Could you check a few things on this model? Use its own coordinates, in mm. A direction names the side the tool comes from. Round coordinates to 2 decimals unless told otherwise and drop trailing zeros. Write each loop counter-clockwise with the first axis right and the second up, starting at its lowest first coordinate (ties: lowest second). Pieces come first, ordered by that corner, then holes. Notation, with made-up numbers: (76.25, 8) -> (93.25, 8) arc R16 ccw to (93.25, 15) -> close; hole circle Ø7 at (89, 83). An arc over 180 degrees is marked (long way). Return JSON: item names as keys, results as strings.
from build123d import *

# Parameters (mm, degrees)
F0_R        = 14.01
F1_DEPTH    = 8.2
F2_T1_DEPTH = 8.2
F3_C1_SIZE  = 1
F3_C2_SIZE  = 1
F3_C3_SIZE  = 1
F3_C4_SIZE  = 1
F3_C5_SIZE  = 1
F3_C6_SIZE  = 1
F3_C7_SIZE  = 1


# Not quite as in the source:
# - a fillet or chamfer that OpenCascade refuses, or shapes differently, is made with other operations: its cross-section is extruded or revolved along the edge and cut away or added


with BuildPart() as f1:
    # F0 (on Top) → F1 (new body)
    with BuildSketch(Plane.XY):
        with BuildLine():
            Line((-22.6979741071, -5), (-18.3303027798, -5))
            ThreePointArc((-18.3303027798, -5), (0, -19), (18.3303027798, -5))
            Line((18.3303027798, -5), (22.6979741071, -5))
            ThreePointArc((22.6979741071, -5), (58.01, 0), (22.6979741071, 5))
            Line((22.6979741071, 5), (18.3303027798, 5))
            ThreePointArc((18.3303027798, 5), (0, 19), (-18.3303027798, 5))
            Line((-18.3303027798, 5), (-22.6979741071, 5))
            ThreePointArc((-22.6979741071, 5), (-58.01, 0), (-22.6979741071, -5))
        make_face()
        with Locations((-40, 0)):
            Circle(F0_R, mode=Mode.SUBTRACT)
        Circle(F0_R, mode=Mode.SUBTRACT)
        with Locations((40, 0)):
            Circle(F0_R, mode=Mode.SUBTRACT)
    extrude(amount=F1_DEPTH)

    # F2: fillet of radius 5 on 8 edges, made by hand

    # F2_s2 → F2_t1 (join)
    with BuildSketch(Plane.XY):
        with BuildLine():
            ThreePointArc((-19.2765808806, -5), (-21.9350728052, -5.7653311007), (-23.7797141095, -7.8270317253))
            ThreePointArc((-23.7797141095, -7.8270317253), (-23.1793468046, -6.4362820074), (-22.6979741071, -5))
            Line((-22.6979741071, -5), (-19.2765808806, -5))
        make_face()
        with BuildLine():
            ThreePointArc((-21.8174242293, -5), (-19.1171156049, -5.7918729423), (-17.2721275148, -7.9166666667))
            ThreePointArc((-17.2721275148, -7.9166666667), (-17.8608509549, -6.4799693801), (-18.3303027798, -5))
            Line((-18.3303027798, -5), (-21.8174242293, -5))
        make_face()
        with BuildLine():
            ThreePointArc((17.2721275148, -7.9166666667), (19.1171156049, -5.7918729423), (21.8174242293, -5))
            Line((21.8174242293, -5), (18.3303027798, -5))
            ThreePointArc((18.3303027798, -5), (17.8608509549, -6.4799693801), (17.2721275148, -7.9166666667))
        make_face()
        with BuildLine():
            ThreePointArc((19.2765808806, -5), (21.9350728052, -5.7653311007), (23.7797141095, -7.8270317253))
            ThreePointArc((23.7797141095, -7.8270317253), (23.1793468046, -6.4362820074), (22.6979741071, -5))
            Line((22.6979741071, -5), (19.2765808806, -5))
        make_face()
        with BuildLine():
            ThreePointArc((21.8174242293, 5), (19.1171156049, 5.7918729423), (17.2721275148, 7.9166666667))
            ThreePointArc((17.2721275148, 7.9166666667), (17.8608509549, 6.4799693801), (18.3303027798, 5))
            Line((18.3303027798, 5), (21.8174242293, 5))
        make_face()
        with BuildLine():
            ThreePointArc((23.7797141095, 7.8270317253), (21.9350728052, 5.7653311007), (19.2765808806, 5))
            Line((19.2765808806, 5), (22.6979741071, 5))
            ThreePointArc((22.6979741071, 5), (23.1793468046, 6.4362820074), (23.7797141095, 7.8270317253))
        make_face()
        with BuildLine():
            ThreePointArc((-17.2721275148, 7.9166666667), (-19.1171156049, 5.7918729423), (-21.8174242293, 5))
            Line((-21.8174242293, 5), (-18.3303027798, 5))
            ThreePointArc((-18.3303027798, 5), (-17.8608509549, 6.4799693801), (-17.2721275148, 7.9166666667))
        make_face()
        with BuildLine():
            ThreePointArc((-19.2765808806, 5), (-21.9350728052, 5.7653311007), (-23.7797141095, 7.8270317253))
            ThreePointArc((-23.7797141095, 7.8270317253), (-23.1793468046, 6.4362820074), (-22.6979741071, 5))
            Line((-22.6979741071, 5), (-19.2765808806, 5))
        make_face()
    extrude(amount=F2_T1_DEPTH)

    # F3: chamfer of 1 on 15 edges, made by hand

    # F3_c1
    f3_c1_edges = [f1.edges().sort_by_distance(p)[0] for p in [
        (0, -19, 8.2),
        (18.6003113726, -6.1724440085, 8.2),
        (-18.6003113726, -6.1724440085, 8.2),
    ]]
    chamfer(f3_c1_edges, length=F3_C1_SIZE)

    # F3_c2
    f3_c2_edges = [f1.edges().sort_by_distance(p)[0] for p in [
        (22.4556214842, -6.1407642155, 8.2),
        (58.01, 0, 8.2),
        (22.4556214842, 6.1407642155, 8.2),
    ]]
    chamfer(f3_c2_edges, length=F3_C2_SIZE)

    # F3_c3
    f3_c3_edges = [f1.edges().sort_by_distance(p)[0] for p in [
        (18.6003113726, 6.1724440085, 8.2),
        (0, 19, 8.2),
        (-18.6003113726, 6.1724440085, 8.2),
    ]]
    chamfer(f3_c3_edges, length=F3_C3_SIZE)

    # F3_c4
    f3_c4_edges = [f1.edges().sort_by_distance(p)[0] for p in [
        (-22.4556214842, 6.1407642155, 8.2),
        (-58.01, 0, 8.2),
        (-22.4556214842, -6.1407642155, 8.2),
    ]]
    chamfer(f3_c4_edges, length=F3_C4_SIZE)

    # F3_c5
    f3_c5_edges = [f1.edges().sort_by_distance(p)[0] for p in [
        (-54.01, 0, 8.2),
    ]]
    chamfer(f3_c5_edges, length=F3_C5_SIZE)

    # F3_c6
    f3_c6_edges = [f1.edges().sort_by_distance(p)[0] for p in [
        (-14.01, 0, 8.2),
    ]]
    chamfer(f3_c6_edges, length=F3_C6_SIZE)

    # F3_c7
    f3_c7_edges = [f1.edges().sort_by_distance(p)[0] for p in [
        (25.99, 0, 8.2),
    ]]
    chamfer(f3_c7_edges, length=F3_C7_SIZE)


solid = f1.part
1) I want a section at A-A, the plane x = 40. Please give me the cut outline in (y, z).
Return value:
{"outline": "(-18.01, 0) -> (-14.01, 0) -> (-14.01, 7.2) -> (-15.01, 8.2) -> (-17.01, 8.2) -> (-18.01, 7.2) -> close; (14.01, 0) -> (18.01, 0) -> (18.01, 7.2) -> (17.01, 8.2) -> (15.01, 8.2) -> (14.01, 7.2) -> close"}
2) I want a section at C-C, the plane y = 0. Please give me the cut outline in (x, z), and give its area (3 significant figures).
Return value:
{"outline": "(-58.01, 0) -> (-54.01, 0) -> (-54.01, 7.2) -> (-55.01, 8.2) -> (-57.01, 8.2) -> (-58.01, 7.2) -> close; (-25.99, 0) -> (-14.01, 0) -> (-14.01, 7.2) -> (-15.01, 8.2) -> (-24.99, 8.2) -> (-25.99, 7.2) -> close; (14.01, 0) -> (25.99, 0) -> (25.99, 7.2) -> (24.99, 8.2) -> (15.01, 8.2) -> (14.01, 7.2) -> close; (54.01, 0) -> (58.01, 0) -> (58.01, 7.2) -> (57.01, 8.2) -> (55.01, 8.2) -> (54.01, 7.2) -> close", "area": "258 mm²"}
3) For faces 1 (the face through (-22.43, -6.12, 3.55)), 2 (the face through (53.363, 4.208, 3.55)), 3 (the face through (18.624, 6.153, 3.55)), which set-ups out of +Z, -Z, +X, -X, +Y, -Y let a thin tool reach every point of the face, with its end or its side?
Return value:
{"face 1": "+Z, -Z, -Y", "face 2": "+Z, -Z", "face 3": "+Z, -Z, +Y"}
4) I want a section at B-B, the plane z = 6. Please give me the cut outline in (x, y).
Return value:
{"outline": "(-23.78, -7.83) arc R5 cw to (-20.55, -5.16) arc R5 cw to (-17.27, -7.92) arc R19 ccw to (17.27, -7.92) arc R5 cw to (20.55, -5.16) arc R5 cw to (23.78, -7.83) arc R18.01 ccw (long way) to (23.78, 7.83) arc R5 cw to (20.55, 5.16) arc R5 cw to (17.27, 7.92) arc R19 ccw to (-17.27, 7.92) arc R5 cw to (-20.55, 5.16) arc R5 cw to (-23.78, 7.83) arc R18.01 ccw (long way) to start; hole circle Ø28.02 at (-40, 0); hole circle Ø28.02 at (0, 0); hole circle Ø28.02 at (40, 0)"}
5) If I drill on probe 1 along Y at (x, z) = (0.5, 1.5); probe 2 along X at (y, z) = (2, 5.5); probe 3 along X at (y, z) = (5, 6.5), over which ranges is the centre line in solid material (lowest first)? Write a range as [from, to].
Return value:
{"probe 1": "[-18.99, -14], [14, 18.99]", "probe 2": "[-57.9, -53.87], [-26.13, -13.87], [13.87, 26.13], [53.87, 57.9]", "probe 3": "[-57.3, -53.09], [-26.91, -13.09], [13.09, 26.91], [53.09, 57.3]"}
6) I want a section at D-D, the plane x = 0. Please give me the cut outline in (y, z), and give its area (3 significant figures).
Return value:
{"outline": "(-19, 0) -> (-14.01, 0) -> (-14.01, 7.2) -> (-15.01, 8.2) -> (-18, 8.2) -> (-19, 7.2) -> close; (14.01, 0) -> (19, 0) -> (19, 7.2) -> (18, 8.2) -> (15.01, 8.2) -> (14.01, 7.2) -> close", "area": "79.8 mm²"}
7) Will these pins go through, and if not, where does the flat tip stop? pin 1 Ø1 at (y, z) = (6.5, 7) entering from -X; pin 2 Ø1 at (x, z) = (15.5, 6.5) entering from -Y; pin 3 Ø4 at (x, y) = (4.5, -11.5) entering from +Z.
Return value:
{"pin 1": "x = -56.98", "pin 2": "y = -11.66", "pin 3": "z = 7.54"}
8) Thinking about a two-plate mould opening in X: for faces 4 (the face through (-18.58, 6.19, 3.55)), 5 (the face through (13, -8, 8.2)), 6 (the face through (18.58, -6.19, 3.55)), which applies, pulls with the +X half, pulls with the -X half, needs draft (parallel to the pull), parting line crosses it, or undercut?
Return value:
{"face 4": "undercut", "face 5": "needs draft", "face 6": "undercut"}
